from build123d import *

# Parameters (mm, degrees)
F1_DEPTH = 1400
F3_R     = 3
F4_D     = 10
F4_DEPTH = 3000


with BuildPart() as f1:
    # F0 (on Front) → F1 (new body)
    with BuildSketch(Plane.XZ):
        Polygon((305.5, 0), (0, 0), (-305.5, 0), (-305.5, -40), (-300, -40), (-300, -5.5), (0, -5.5), (300, -5.5), (300, -14.070651), (300, -40), (305.5, -40), align=None)
    extrude(amount=F1_DEPTH)

    # F3
    f3_edges = [f1.edges().sort_by_distance(p)[0] for p in [
        (-305.5, -700, 0),
        (305.5, -700, 0),
    ]]
    fillet(f3_edges, radius=F3_R)

    # F4
    with Locations(Plane(origin=(-305.5, 0, 0), x_dir=(0, -1, 0), z_dir=(-1, 0, 0))):
        with Locations((100, -25.5), (700, -25.5), (1300, -25.5)):
            Hole(F4_D / 2, depth=F4_DEPTH)


solid = f1.part
Geometry: final body of the model. Coordinates: model frame, mm. A direction names the side the tool comes from. Round coordinates to 2 decimals unless told otherwise and drop trailing zeros. Write each loop counter-clockwise with the first axis right and the second up, starting at its lowest first coordinate (ties: lowest second). Pieces come first, ordered by that corner, then holes. Notation, with made-up numbers: M 59,4 L 78,4 A31 cw 78,40 Z; hole C -29,-37.5 d1. An arc over 180 degrees is marked long. Write item = value, one per line.
Item 1: Material intervals for line 1 along Y through (x, z) = (-301, -25); line 2 along X through (y, z) = (-837.5, -30); line 3 along Z through (x, y) = (-302.05, -700), sorted ascending. Write a range as [from, to].
Findings:
line_1 = [-1400, -1304.97], [-1295.03, -704.97], [-695.03, -104.97], [-95.03, 0]
line_2 = [-305.5, -300], [300, 305.5]
line_3 = [-40, -30.5], [-20.5, 0]
Item 2: Pin query (flat end, axial travel): P1, Ø13, axis at y = -100, z = -25.5, coming from the +X side; P2, Ø8, axis at x = -50.5, y = -623.5, coming from the -Z side. Return the tip coordinate at first contact, or that it passes through.
Findings:
P1 = 305.5
P2 = -5.5
Item 3: Section query C-C on x = -172. Return loops of the section in (y, z).
Findings:
outline = M -1400,-5.5 L 0,-5.5 L 0,0 L -1400,0 Z
Item 4: Pull-direction query (X, two-part tool) for faces 1 (the face through (300, -690, -23)), 2 (the face through (305.5, -690, -22)), 3 (the face through (4, -690, 0)); classes: pulls with the +X half, pulls with the -X half, needs draft (parallel to the pull), parting line crosses it, or undercut.
Findings:
face_1 = undercut
face_2 = pulls with the +X half
face_3 = needs draft
Item 5: Section query A-A on z = -14. Return loops of the section in (x, y).
Findings:
outline = M -305.5,-1400 L -300,-1400 L -300,0 L -305.5,0 Z; M 300,-1400 L 305.5,-1400 L 305.5,0 L 300,0 Z
Item 6: Section query B-B on y = -1171. Return loops of the section in (x, z).
Findings:
outline = M -305.5,-40 L -300,-40 L -300,-5.5 L 300,-5.5 L 300,-40 L 305.5,-40 L 305.5,-3 A3 ccw 302.5,0 L -302.5,0 A3 ccw -305.5,-3 Z
Item 7: Access query for faces 4 (the face through (-300, -690, -23)), 5 (the face through (-1, -1400, -2)). Directions: +Z, -Z, +X, -X, +Y, -Y. A direction counts if a zero-diameter tool reaches every point of the face in a straight line with its end or side. Return the directions, or none.
Findings:
face_4 = -Z, +Y, -Y
face_5 = +Z, -Z, +X, -X, -Y
